Build history of the part. All positions in model axes, mm. A direction names the side the tool comes from. Give positions to 0.01 mm unless a question says otherwise; leave off trailing zeros. Write each loop counter-clockwise with the first axis right and the second up, starting at its lowest first coordinate (ties: lowest second). Pieces come first, ordered by that corner, then holes. Notation, with made-up numbers: (40.25, -3) - (90.25, -3) arc R30 cw to (90.25, 25) - close; hole circle Ø4 at (73.5, 41). An arc over 180 degrees is marked (long way). Use one line per item in the form item = value. Start each with the question number.
from build123d import *

# Parameters (mm, degrees)
CROQUIS1_R                          = 7
SALIENTE_EXTRUIR1_DEPTH             = 25
CROQUIS2_R                          = 2.5
CORTAR_EXTRUIR1_DEPTH               = 12.5
CROQUIS3_R                          = 4
CORTAR_EXTRUIR2_DEPTH               = 12.5
CHAFL_N1_SIZE                       = 1
CHAFL_N2_SIZE                       = 1
TALADRO_DE_MARGEN_PARA_M1_41_REACH  = 27.44
TALADRO_DE_MARGEN_PARA_M1_41_BORE_R = 0.8
TALADRO_DE_MARGEN_PARA_M1_42_REACH  = 27.426
TALADRO_DE_MARGEN_PARA_M1_42_BORE_R = 0.8


with BuildPart() as part:
    # Croquis1 → Saliente-Extruir1 (new body)
    with BuildSketch(Plane(origin=(0, 0, 0), x_dir=(0, 0, -1), z_dir=(1, 0, 0))):
        Circle(CROQUIS1_R)
    extrude(amount=SALIENTE_EXTRUIR1_DEPTH)

    # Croquis2 → Cortar-Extruir1 (cut)
    with BuildSketch(Plane(origin=(25, 0, 0), x_dir=(0, 0, -1), z_dir=(1, 0, 0))):
        Circle(CROQUIS2_R)
    extrude(amount=-CORTAR_EXTRUIR1_DEPTH, mode=Mode.SUBTRACT)

    # Croquis3 → Cortar-Extruir2 (cut)
    with BuildSketch(Plane.ZY):
        Circle(CROQUIS3_R)
    extrude(amount=-CORTAR_EXTRUIR2_DEPTH, mode=Mode.SUBTRACT)

    # Chaflán1
    chafl_n1_edges = [part.edges().sort_by_distance(p)[0] for p in [
        (25, 0, 7),
    ]]
    chamfer(chafl_n1_edges, length=CHAFL_N1_SIZE)

    # Chaflán2
    chafl_n2_edges = [part.edges().sort_by_distance(p)[0] for p in [
        (0, 0, 7),
    ]]
    chamfer(chafl_n2_edges, length=CHAFL_N2_SIZE)

    # Taladro de margen para M1.41 bore (on position points) → Taladro de margen para M1.41 (cut, up to next)
    with BuildSketch(Plane(origin=(5, 6.998215778, -0.158037721), x_dir=(0, 0.022576817235, 0.999745111178), z_dir=(0, 0.999745111178, -0.022576817235)), mode=Mode.PRIVATE) as taladro_de_margen_para_m1_41_sk1:
        Circle(TALADRO_DE_MARGEN_PARA_M1_41_BORE_R)
    taladro_de_margen_para_m1_41_tool1 = extrude(taladro_de_margen_para_m1_41_sk1.sketch, amount=-TALADRO_DE_MARGEN_PARA_M1_41_REACH, mode=Mode.PRIVATE) & part.part
    add(taladro_de_margen_para_m1_41_tool1.solids().sort_by_distance((5, 6.998216, -0.158038))[0], mode=Mode.SUBTRACT)

    # Taladro de margen para M1.42 bore (on position points) → Taladro de margen para M1.42 (cut, up to next)
    with BuildSketch(Plane(origin=(20, 6.999207069, -0.10535848), x_dir=(0, 0.01505121149, 0.999886724101), z_dir=(0, 0.999886724101, -0.01505121149)), mode=Mode.PRIVATE) as taladro_de_margen_para_m1_42_sk1:
        Circle(TALADRO_DE_MARGEN_PARA_M1_42_BORE_R)
    taladro_de_margen_para_m1_42_tool1 = extrude(taladro_de_margen_para_m1_42_sk1.sketch, amount=-TALADRO_DE_MARGEN_PARA_M1_42_REACH, mode=Mode.PRIVATE) & part.part
    add(taladro_de_margen_para_m1_42_tool1.solids().sort_by_distance((20, 6.999207, -0.105358))[0], mode=Mode.SUBTRACT)


solid = part.part
(1) Cut at B-B, the plane x = 8.75. Give the cut face in (y, z).
(2) Cut at C-C, the plane z = 0. State how many separate pieces and enclosed holes the cut face has, then the cut area to 3 significant figures.
(3) Which spindle directions (+Z, -Z, +X, -X, +Y, -Y) get a long thin tool onto all of the face, cutting with end or side? Do faces 4 (the cylindrical face through (4.22, 5.47, -0.3)), 5 (the flat face through (25, 0, -3)), 6 (the flat face through (12.5, 2, 2)). Say none if no direction does.
(4) Pin check, flat tip, straight feed: pin 1 Ø5 at (x, z) = (5, -3.5) entering from +Y. Stop position of the tip, or through.
(5) Two-plate mould, pull along Z, no slides. Class faces 1 (the cylindrical face through (6.162, -3.905, -0.867)), 2 (the flat face through (0, -3.92, 1.42)), 3 (the cylindrical face through (12.339, -2.681, -6.466)): +Z half, -Z half, draft (parallel to the pull), parting line (faces both ways), or undercut.
(6) Wall check: line 1 (Y direction, x = 9.25, z = 0); line 2 (Y direction, x = 20.5, z = -1.25); line 3 (X direction, y = 1, z = 3). Give the ranges that are in metal, low to high. Write a range as from..to.
(7) Cut at A-A, the plane y = 0. Give the cut face in (x, z).
Solution:
q1.outline = circle Ø14 at (0, 0); hole circle Ø8 at (0, 0)
q2.separate_pieces = 4
q2.enclosed_holes = 0
q2.area = 174 mm2
q3.face_4 = none
q3.face_5 = +Z, -Z, +X, +Y, -Y
q3.face_6 = -X
q4.pin_1 = 6.93
q5.face_1 = undercut
q5.face_2 = draft
q5.face_3 = parting line
q6.line_1 = -7..-4, 4..7
q6.line_2 = -6.89..-2.17, 2.17..6.89
q6.line_3 = 12.5..25
q7.outline = (0, -6) - (1, -7) - (24, -7) - (25, -6) - (25, -2.5) - (12.5, -2.5) - (12.5, -4) - (0, -4) - close; (0, 4) - (12.5, 4) - (12.5, 2.5) - (25, 2.5) - (25, 6) - (24, 7) - (1, 7) - (0, 6) - close
